Could you check a few things on this model? Use its own coordinates, in mm. A direction names the side the tool comes from. Give positions to 0.01 mm unless a question says otherwise; leave off trailing zeros. Loops run counter-clockwise (first coordinate to the right, second up) from the corner with the lowest first, then second, coordinate; pieces in that order, holes last. Notation, with made-up numbers: (25.25, 72) -> (48.25, 72) arc R14 ccw to (48.25, 76) -> close; hole circle Ø5 at (-29.75, 54.5). An arc over 180 degrees is marked (long way). Write each question's results on one line, items separated by ' | '. Start each with the question number.
Q1. Will these pins go through, and if not, where does the flat tip stop? P1, Ø20.5, axis at y = 133.5, z = 33, coming from the -X side; P2, Ø12, axis at y = 36.5, z = 14.5, coming from the +X side; P3, Ø12, axis at x = -7.5, z = 28.5, coming from the +Y side.
Q2. If we section it at B-B, the plane y = 59: List the corners of the cut face in (x, z) for me, plus the area to 3 significant figures.
Q3. Which directions (+Z, -Z, +X, -X, +Y, -Y) give clear straight access to the entire face, cutting with the end or side of a thin tool? Please do faces 4 (the face through (-20.5, 0, 22)), 5 (the face through (0.55, 104.19, 46.38)), 6 (the face through (-2, 70, 35)).
Q4. We'd pull the mould along Y, two halves only. Please class faces 1 (the face through (0.1, 173.7, -23.8)), 2 (the face through (0.52, 130.39, 5.39)), 3 (the face through (-2, 98.932, 27)): released by +Y, released by -Y, zero draft, split by the parting line, or undercut.
Q5. If we section it at C-C, the plane z = 23.5: List the corners of the cut face in (x, y) for me, plus the area to 3 significant figures.
Q6. If I drill on line 1 along X through (y, z) = (15.5, 30); line 2 along Z through (x, y) = (-24, -16); line 3 along X through (y, z) = (210, 51), over which ranges is the centre line in solid material (lowest first)?
Q7. If we section it at A-A, the plane y = 0: List the corners of the cut face in (x, z) for me.
from build123d import *

# Parameters (mm, degrees)
BOSS_EXTRUDE1_DEPTH     = 55
CUT_EXTRUDE3_DEPTH      = 28
CUT_EXTRUDE4_DEPTH      = 40.029131656
CUT_EXTRUDE4_DEPTH_BACK = 40.029131656
SKETCH18_R              = 4.5
SKETCH18_R_2            = 3
CUT_EXTRUDE5_DEPTH      = 24.598674983
CUT_EXTRUDE5_DEPTH_BACK = 28
CUT_EXTRUDE6_DEPTH      = 26.134831719
CUT_EXTRUDE6_DEPTH_BACK = 85.175442033
SKETCH21_R              = 4
CUT_EXTRUDE7_DEPTH      = 25.226187847
CUT_EXTRUDE7_DEPTH_BACK = 56.443633682
SKETCH22_W              = 31
SKETCH22_H              = 66
CUT_EXTRUDE8_DEPTH      = 34
SKETCH30_R              = 3.775
BOSS_EXTRUDE2_DEPTH     = 30
CUT_EXTRUDE9_START      = 20
CUT_EXTRUDE9_DEPTH      = 15


with BuildPart() as part:
    # Sketch1 → Boss-Extrude1 (new body)
    with BuildSketch(Plane.XY):
        with BuildLine():
            Line((-22.827528122, 39.292617223), (-38.880054689, 170.029954628))
            ThreePointArc((-38.880054689, 170.029954628), (-36.535345881, 182.138559801), (-27.533199801, 190.569297881))
            ThreePointArc((-27.533199801, 190.569297881), (-19.660174006, 198.055084384), (-16.79086128, 208.533088928))
            ThreePointArc((-16.79086128, 208.533088928), (0, 226.212902341), (16.79086128, 208.533088928))
            ThreePointArc((16.79086128, 208.533088928), (19.660174006, 198.055084384), (27.533199801, 190.569297881))
            ThreePointArc((27.533199801, 190.569297881), (36.535345881, 182.138559801), (38.880054689, 170.029954628))
            Line((38.880054689, 170.029954628), (22.827528122, 39.292617223))
            ThreePointArc((22.827528122, 39.292617223), (23.667809595, 30.306601974), (27.215074691, 22.007719318))
            ThreePointArc((27.215074691, 22.007719318), (0, -35), (-27.215074691, 22.007719318))
            ThreePointArc((-27.215074691, 22.007719318), (-23.667809595, 30.306601974), (-22.827528122, 39.292617223))
        make_face()
    extrude(amount=BOSS_EXTRUDE1_DEPTH)

    # Sketch5 → Cut-Extrude3 (cut)
    with BuildSketch(Plane.XY):
        Polygon((16.97, -20.5), (-16.97, -20.5), (-20.5, -16.97), (-20.5, 16.97), (-16.97, 20.5), (16.97, 20.5), (20.5, 16.97), (20.5, -16.97), align=None)
    extrude(amount=CUT_EXTRUDE3_DEPTH, mode=Mode.SUBTRACT)

    # Sketch15 → Cut-Extrude4 (cut, two sides)
    with BuildSketch(Plane(origin=(0, 0, 0), x_dir=(0, 0, -1), z_dir=(1, 0, 0))) as cut_extrude4_sk:
        Polygon((-38, -35), (-38, 30.17907071), (-55, 180.299626254), (-55, -35), align=None)
        Polygon((-4.401325017, 156.123614829), (-12.400064416, 226.757450259), (0, 226.212902341), (0, 149.914783233), (0, 117.257182084), (0, -35), (-17, -35), (-17, 30.65016827), (-6.349536626, 105.369192589), align=None)
    extrude(amount=CUT_EXTRUDE4_DEPTH, mode=Mode.SUBTRACT)
    extrude(cut_extrude4_sk.sketch, amount=-CUT_EXTRUDE4_DEPTH_BACK, mode=Mode.SUBTRACT)

    # Sketch18 → Cut-Extrude5 (cut, two sides)
    with BuildSketch(Plane(origin=(0, 0, 28), x_dir=(-1, 0, 0), z_dir=(0, 0, -1))) as cut_extrude5_sk:
        Circle(SKETCH18_R)
        with Locations((-15.199466094, 15.199466094)):
            Circle(SKETCH18_R_2)
        with Locations((15.199466094, 15.199466094)):
            Circle(SKETCH18_R_2)
        with Locations((15.199466094, -15.199466094)):
            Circle(SKETCH18_R_2)
        with Locations((-15.199466094, -15.199466094)):
            Circle(SKETCH18_R_2)
    extrude(amount=CUT_EXTRUDE5_DEPTH, mode=Mode.SUBTRACT)
    extrude(cut_extrude5_sk.sketch, amount=-CUT_EXTRUDE5_DEPTH_BACK, mode=Mode.SUBTRACT)

    # Sketch20 → Cut-Extrude6 (cut, two sides)
    with BuildSketch(Plane(origin=(-17.735618329, -2.177660109, 0), x_dir=(0, 0, 1), z_dir=(-0.992546152, -0.121869343, 0))) as cut_extrude6_sk:
        Polygon((16.527188649, 200.652068787), (48.527188649, 200.652068787), (51.520800543, 224.652068787), (19.520800543, 224.652068787), align=None)
    extrude(amount=CUT_EXTRUDE6_DEPTH, mode=Mode.SUBTRACT)
    extrude(cut_extrude6_sk.sketch, amount=-CUT_EXTRUDE6_DEPTH_BACK, mode=Mode.SUBTRACT)

    # Sketch21 → Cut-Extrude7 (cut, two sides)
    with BuildSketch(Plane(origin=(0, -3.866612347, 34.144587862), x_dir=(1, 0, 0), z_dir=(0, -0.11252313, 0.993649106))) as cut_extrude7_sk:
        with Locations((0, 220.965020256)):
            Circle(SKETCH21_R)
    extrude(amount=CUT_EXTRUDE7_DEPTH, mode=Mode.SUBTRACT)
    extrude(cut_extrude7_sk.sketch, amount=-CUT_EXTRUDE7_DEPTH_BACK, mode=Mode.SUBTRACT)

    # Sketch22 → Cut-Extrude8 (cut)
    with BuildSketch(Plane(origin=(0, -3.866612347, 34.144587862), x_dir=(1, 0, 0), z_dir=(0, -0.11252313, 0.993649106))):
        with Locations((0, 149.850276465)):
            Rectangle(SKETCH22_W, SKETCH22_H)
    extrude(amount=-CUT_EXTRUDE8_DEPTH, mode=Mode.SUBTRACT)

    # Sketch30 → Boss-Extrude2 (add)
    with BuildSketch(Plane(origin=(0, 1.484646511, -13.110350529), x_dir=(-1, 0, 0), z_dir=(0, 0.11252313, -0.993649106))):
        with Locations((0, 169.857341116)):
            Circle(SKETCH30_R)
    extrude(amount=BOSS_EXTRUDE2_DEPTH)

    # Sketch31 → Cut-Extrude9 (cut)
    with BuildSketch(Plane.XY.offset(CUT_EXTRUDE9_START)):
        Polygon((-16.71237329, 40.092398344), (-23.538465204, 98.932300939), (19.683150051, 98.932300939), (14.908186254, 40.092398344), align=None)
    extrude(amount=CUT_EXTRUDE9_DEPTH, mode=Mode.SUBTRACT)


solid = part.part
Final values:
1) P1: stops at x = -35.65 | P2: stops at x = 23.5 | P3: stops at y = 201.97
2) outline: (-25.25, 12.96) -> (25.25, 12.96) -> (25.25, 41.26) -> (-25.25, 41.26) -> close; hole (-18.91, 20) -> (16.44, 20) -> (16.44, 35) -> (-18.91, 35) -> close | area: 899 mm²
3) face 4: -Z | face 5: +Z, +X, -X, -Y | face 6: none
4) face 1: released by +Y | face 2: released by -Y | face 3: undercut
5) outline: (-38.88, 170.03) -> (-22.83, 39.29) arc R29.17 cw to (-27.22, 22.01) arc R35 ccw (long way) to (27.22, 22.01) arc R29.17 cw to (22.83, 39.29) -> (38.88, 170.03) arc R20 ccw to (27.53, 190.57) arc R20.24 cw to (17.22, 204.27) -> (-18.7, 199.86) arc R20.24 cw to (-27.53, 190.57) arc R20 ccw to start; hole (-23.54, 98.93) -> (-16.71, 40.09) -> (14.91, 40.09) -> (19.68, 98.93) -> close; hole (-20.5, -16.97) -> (-16.97, -20.5) -> (16.97, -20.5) -> (20.5, -16.97) -> (20.5, 16.97) -> (16.97, 20.5) -> (-16.97, 20.5) -> (-20.5, 16.97) -> close; hole (-15.5, 114.94) -> (15.5, 114.94) -> (15.5, 181.36) -> (-15.5, 181.36) -> close | area: 8,320 mm²
6) line 1: x = -31.38 to -18.18, -12.21 to 12.21, 18.18 to 31.38 | line 2: z = 17 to 38 | line 3: x = -16.8 to 16.8
7) outline: (-35, 17) -> (-20.5, 17) -> (-20.5, 28) -> (-4.5, 28) -> (-4.5, 38) -> (-35, 38) -> close; (4.5, 28) -> (20.5, 28) -> (20.5, 17) -> (35, 17) -> (35, 38) -> (4.5, 38) -> close
